Can you work these out from the model? Positions are in its coordinate system, mm. Round coordinates to 2 decimals unless told otherwise and drop trailing zeros. Loops run counter-clockwise (first coordinate to the right, second up) from the corner with the lowest first, then second, coordinate; pieces in that order, holes last. Notation, with made-up numbers: (13, 62.5) -> (53, 62.5) arc R8 ccw to (53, 70.5) -> close; hole circle Ø9 at (65.5, 38). An arc over 180 degrees is marked (long way). Write each question's results on one line, items separated by ' | '.
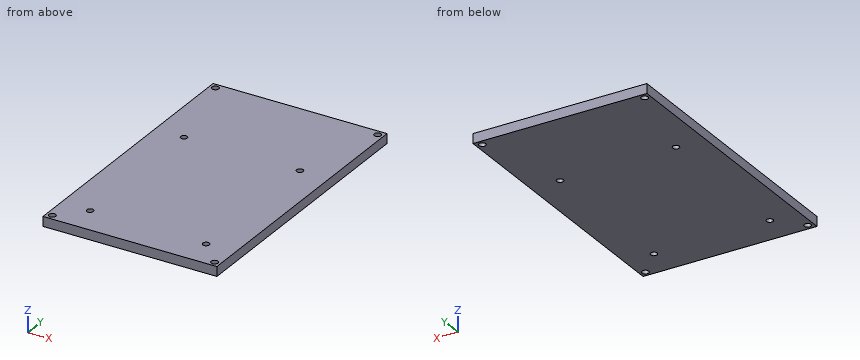
from build123d import *

# Parameters (mm, degrees)
SKETCH1_W           = 90
SKETCH1_H           = 145
BOSS_EXTRUDE1_DEPTH = 5
SKETCH2_R           = 1.75
CUT_EXTRUDE1_DEPTH  = 86.476604986
SKETCH3_R           = 1.7
CUT_EXTRUDE2_DEPTH  = 86.476604986


with BuildPart() as part:
    # Sketch1 → Boss-Extrude1 (new body)
    with BuildSketch(Plane.XY):
        Rectangle(SKETCH1_W, SKETCH1_H)
    extrude(amount=BOSS_EXTRUDE1_DEPTH)

    # Sketch2 → Cut-Extrude1 (cut, through all)
    with BuildSketch(Plane(origin=(0, 0, 0), x_dir=(-1, 0, 0), z_dir=(0, 0, -1))):
        with Locations((-42, 69.5)):
            Circle(SKETCH2_R)
        with Locations(Location((-42, -69.5, 0), (0, 0, 180))):
            Circle(SKETCH2_R)
        with Locations(Location((42, 69.5, 0), (0, 0, 180))):
            Circle(SKETCH2_R)
        with Locations((42, -69.5)):
            Circle(SKETCH2_R)
    extrude(amount=-CUT_EXTRUDE1_DEPTH, mode=Mode.SUBTRACT)

    # Sketch3 → Cut-Extrude2 (cut, through all)
    with BuildSketch(Plane(origin=(0, 0, 0), x_dir=(-1, 0, 0), z_dir=(0, 0, -1))):
        with Locations((-30, 23)):
            Circle(SKETCH3_R)
        with Locations(Location((30, 23, 0), (0, 0, 180))):
            Circle(SKETCH3_R)
        with Locations((30, -57)):
            Circle(SKETCH3_R)
        with Locations(Location((-30, -57, 0), (0, 0, 180))):
            Circle(SKETCH3_R)
    extrude(amount=-CUT_EXTRUDE2_DEPTH, mode=Mode.SUBTRACT)


solid = part.part
1. Please list where these lines run through material, in increasing order: line 1 (Y direction, x = -42, z = 1.65); line 2 (Y direction, x = -30, z = 3.6); line 3 (X direction, y = 69.5, z = 2.9). Write a range as from..to.
Final values:
line 1: -72.5..-71.25, -67.75..67.75, 71.25..72.5 | line 2: -72.5..-58.7, -55.3..21.3, 24.7..72.5 | line 3: -45..-43.75, -40.25..40.25, 43.75..45
2. If we section it at B-B (y = 69.5): List the corners of the cut face in (x, z) for me, then the cut area to 3 significant figures.
Final values:
outline: (-45, 0) -> (-43.75, 0) -> (-43.75, 5) -> (-45, 5) -> close; (-40.25, 0) -> (40.25, 0) -> (40.25, 5) -> (-40.25, 5) -> close; (43.75, 0) -> (45, 0) -> (45, 5) -> (43.75, 5) -> close | area: 415 mm2
3. Will this pin go through, and if not, where does the flat tip stop? pin 1 (4 mm diameter, centred on x = -30, y = -57, fed in from -Z).
Final values:
pin 1: z = 0
4. If we section it at A-A (x = -42): List the corners of the cut face in (y, z) for me, then the cut area to 3 significant figures.
Final values:
outline: (-72.5, 0) -> (-71.25, 0) -> (-71.25, 5) -> (-72.5, 5) -> close; (-67.75, 0) -> (67.75, 0) -> (67.75, 5) -> (-67.75, 5) -> close; (71.25, 0) -> (72.5, 0) -> (72.5, 5) -> (71.25, 5) -> close | area: 690 mm2
